```python
from build123d import *

# Parameters (mm, degrees)
SKETCH1_W                                      = 85
SKETCH1_H                                      = 85
BOSS_EXTRUDE1_DEPTH                            = 3
FILLET1_R                                      = 10
CUT_EXTRUDE1_REACH                             = 5
SKETCH3_W                                      = 25
SKETCH3_H                                      = 25
CSK_FOR_M3_FLAT_HEAD_MACHINE_SCREW1_AT_2_COUNT = 2
CSK_FOR_M3_FLAT_HEAD_MACHINE_SCREW1_AT_2_PITCH = 65
CSK_FOR_M3_FLAT_HEAD_MACHINE_SCREW1_AT_3_COUNT = 2
CSK_FOR_M3_FLAT_HEAD_MACHINE_SCREW1_AT_3_PITCH = 91.923881554
CSK_FOR_M3_FLAT_HEAD_MACHINE_SCREW1_AT_4_COUNT = 2
CSK_FOR_M3_FLAT_HEAD_MACHINE_SCREW1_AT_4_PITCH = 65
SKETCH6_R                                      = 1
CUT_EXTRUDE2_DEPTH                             = 4


with BuildPart() as part:
    # Sketch1 → Boss-Extrude1 (new body)
    with BuildSketch(Plane(origin=(0, 0, 0), x_dir=(1, 0, 0), z_dir=(0, 1, 0))):
        Rectangle(SKETCH1_W, SKETCH1_H)
    extrude(amount=BOSS_EXTRUDE1_DEPTH)

    # Fillet1
    fillet1_edges = [part.edges().sort_by_distance(p)[0] for p in [
        (42.5, 1.5, 42.5),
        (-42.5, 1.5, 42.5),
        (-42.5, 1.5, -42.5),
        (42.5, 1.5, -42.5),
    ]]
    fillet(fillet1_edges, radius=FILLET1_R)

    # Sketch3 → Cut-Extrude1 (cut, up to next)
    with BuildSketch(Plane(origin=(0, 3, 0), x_dir=(1, 0, 0), z_dir=(0, 1, 0)), mode=Mode.PRIVATE) as cut_extrude1_sk1:
        Rectangle(SKETCH3_W, SKETCH3_H)
    cut_extrude1_tool1 = extrude(cut_extrude1_sk1.sketch, amount=-CUT_EXTRUDE1_REACH, mode=Mode.PRIVATE) & part.part
    add(cut_extrude1_tool1.solids().sort_by_distance((0, 3, 0))[0], mode=Mode.SUBTRACT)

    # Sketch4 → CSK for M3 Flat Head Machine Screw1 (revolve, cut)
    with BuildSketch(Plane(origin=(32.5, 3, -32.5), x_dir=(0, 0, 1), z_dir=(1, 0, 0))):
        Polygon((0, 0), (0, 3), (1.6, 3), (1.6, 1.7), (3.15, 0.15), (3.15, 0), align=None)
    csk_for_m3_flat_head_machine_screw1 = revolve(axis=Axis((32.5, 9.35, -32.5), (0, -1, 0)), mode=Mode.SUBTRACT)

    # CSK for M3 Flat Head Machine Screw1 at 2: CSK for M3 Flat Head Machine Screw1 ×2
    with Locations(*[(0, 0, i * CSK_FOR_M3_FLAT_HEAD_MACHINE_SCREW1_AT_2_PITCH) for i in range(1, CSK_FOR_M3_FLAT_HEAD_MACHINE_SCREW1_AT_2_COUNT)]):
        add(csk_for_m3_flat_head_machine_screw1, mode=Mode.SUBTRACT)

    # CSK for M3 Flat Head Machine Screw1 at 3: CSK for M3 Flat Head Machine Screw1 ×2
    with Locations(*[Vector(-0.707106781, 0, 0.707106781) * (i * CSK_FOR_M3_FLAT_HEAD_MACHINE_SCREW1_AT_3_PITCH) for i in range(1, CSK_FOR_M3_FLAT_HEAD_MACHINE_SCREW1_AT_3_COUNT)]):
        add(csk_for_m3_flat_head_machine_screw1, mode=Mode.SUBTRACT)

    # CSK for M3 Flat Head Machine Screw1 at 4: CSK for M3 Flat Head Machine Screw1 ×2
    with Locations(*[(-i * CSK_FOR_M3_FLAT_HEAD_MACHINE_SCREW1_AT_4_PITCH, 0, 0) for i in range(1, CSK_FOR_M3_FLAT_HEAD_MACHINE_SCREW1_AT_4_COUNT)]):
        add(csk_for_m3_flat_head_machine_screw1, mode=Mode.SUBTRACT)

    # Sketch6 → Cut-Extrude2 (cut, through all)
    with BuildSketch(Plane(origin=(0, 3, 0), x_dir=(1, 0, 0), z_dir=(0, 1, 0))):
        with Locations((-14.5, 14.5)):
            Circle(SKETCH6_R)
        with Locations((14.5, 14.5)):
            Circle(SKETCH6_R)
        with Locations((14.5, -14.5)):
            Circle(SKETCH6_R)
        with Locations((-14.5, -14.5)):
            Circle(SKETCH6_R)
    extrude(amount=-CUT_EXTRUDE2_DEPTH, mode=Mode.SUBTRACT)


solid = part.part
```
The model under review builds one solid part; all positions refer to its coordinate system, in mm. A direction names the side the tool comes from. Coordinates: 2 decimals unless noted, no trailing zeros. Write each loop counter-clockwise with the first axis right and the second up, starting at its lowest first coordinate (ties: lowest second). Pieces come first, ordered by that corner, then holes.
1) We need section A-A on z = 8. State the section outline as (x, y) points, then the cut area to 3 significant figures.
2) We need section B-B on y = 1.8. Count the separate pieces of the cut face and the enclosed holes in it, then the cut area to 3 significant figures.
3) To check wall thickness, follow probe 1 along X at (y, z) = (0.8, 32.5); probe 2 along Z at (x, y) = (6, 1.85). State the ranges of each line that lie inside material, in increasing order.
4) The part is to be moulded in two halves that separate along Z. For faces 3 (the face through (0, 1, -42.5)), 4 (the face through (0, 2, 12.5)), 5 (the face through (0, 1, 42.5)), say which applies: pulls with the +Z half, pulls with the -Z half, needs draft (parallel to the pull), parting line crosses it, or undercut.
5) Machinability: for faces 1 (the face through (0, 2, -12.5)), 2 (the face through (-39.65, 1.52, 39.49)), which of the approach directions +Z, -Z, +X, -X, +Y, -Y give a long, thin tool a straight path to every point of the face, cutting with its end or side? Answer none if there is none.
6) We need section D-D on x = 9. State the section outline as (y, z) points.
7) Clearance check with flat-ended pins moving along their axes: pin 1 Ø1.2 at (x, z) = (-14.5, 14.5) entering from -Y; pin 2 Ø3.5 at (x, z) = (32.5, 32.5) entering from +Y; pin 3 Ø5 at (x, z) = (32.5, 32.5) entering from +Y. State where each tip first meets the part, or that it passes through.
8) We need section C-C on x = -14.5. State the section outline as (y, z) points.
Answer list:
1. outline: (-42.5, 0) - (-12.5, 0) - (-12.5, 3) - (-42.5, 3) - close; (12.5, 0) - (42.5, 0) - (42.5, 3) - (12.5, 3) - close
1. area: 180 mm2
2. separate pieces: 1
2. enclosed holes: 9
2. area: 6,450 mm2
3. probe 1: x = -42.5 to -34.1, -30.9 to 30.9, 34.1 to 42.5
3. probe 2: z = -42.5 to -12.5, 12.5 to 42.5
4. face 3: pulls with the -Z half
4. face 4: undercut
4. face 5: pulls with the +Z half
5. face 1: +Y, -Y
5. face 2: +Z, -X, +Y, -Y
6. outline: (0, -42.5) - (3, -42.5) - (3, -12.5) - (0, -12.5) - close; (0, 12.5) - (3, 12.5) - (3, 42.5) - (0, 42.5) - close
7. pin 1: passes through
7. pin 2: stops at y = 1.45
7. pin 3: stops at y = 2.2
8. outline: (0, -42.5) - (3, -42.5) - (3, -15.5) - (0, -15.5) - close; (0, -13.5) - (3, -13.5) - (3, 13.5) - (0, 13.5) - close; (0, 15.5) - (3, 15.5) - (3, 42.5) - (0, 42.5) - close
